```python
from build123d import *

# Parameters (mm, degrees)
F0_R      = 5.5120501068
F1_DEPTH  = 50
F3_DEPTH  = 13
F4_R      = 10
F5_DEPTH  = 7
F6_R      = 5
F7_DEPTH  = 6
F8_R      = 5.5120501068
F9_DEPTH  = 9
F11_DEPTH = 381
F13_DEPTH = 381
F14_W     = 50
F14_H     = 12
F15_DEPTH = 15
F16_R     = 5
F17_DEPTH = 381


with BuildPart() as f1:
    # F0 (on Front) → F1 (new body)
    with BuildSketch(Plane.XZ):
        with BuildLine():
            Line((60, -15), (60, 0))
            Line((60, 0), (0, 0))
            Line((0, 0), (0, -63))
            Line((0, -63), (45, -63))
            Line((45, -63), (72.4561188247, -53.0067899993))
            ThreePointArc((72.4561188247, -53.0067899993), (74.5109412295, -53.1845320084), (76.2667195414, -54.2667195414))
            Line((76.2667195414, -54.2667195414), (85, -63))
            Line((85, -63), (100, -63))
            Line((100, -63), (100, -15))
            Line((100, -15), (60, -15))
        make_face()
        with Locations((90, -28)):
            Circle(F0_R, mode=Mode.SUBTRACT)
    extrude(amount=F1_DEPTH)

    # F2 (on face) → F3 (cut)
    with BuildSketch(Plane.XZ.offset(50)):
        with BuildLine():
            Line((30, 0), (0, 0))
            Line((0, 0), (0, -50.6242252886))
            ThreePointArc((0, -50.6242252886), (11.1042474662, -53.9150696691), (22.5, -51.8484800354))
            ThreePointArc((22.5, -51.8484800354), (54.7104431454, -31.7939424821), (30, -3))
            Line((30, -3), (30, 0))
        make_face()
    extrude(amount=-F3_DEPTH, mode=Mode.SUBTRACT)

    # F4 (on face) → F5 (join)
    with BuildSketch(Plane.XZ.offset(37)):
        with Locations((30, -28)):
            Circle(F4_R)
    extrude(amount=F5_DEPTH)

    # F6 (on face) → F7 (join)
    with BuildSketch(Plane.XZ.offset(44)):
        with Locations((30, -28)):
            Circle(F6_R)
    extrude(amount=F7_DEPTH)

    # F8 (on face) → F9 (cut)
    with BuildSketch(Plane.XZ.offset(50)):
        with BuildLine():
            Line((100, -15), (80, -15))
            Line((80, -15), (80, -28))
            ThreePointArc((80, -28), (85.8578643763, -42.1421356237), (100, -48))
            Line((100, -48), (100, -15))
        make_face()
        with Locations((90, -28)):
            Circle(F8_R, mode=Mode.SUBTRACT)
    extrude(amount=-F9_DEPTH, mode=Mode.SUBTRACT)

    # F10 (on face) → F11 (cut)
    with BuildSketch(Plane.XZ.offset(50)):
        with BuildLine():
            Line((30, 0), (0, 0))
            Line((0, 0), (0, -56.8121126443))
            ThreePointArc((0, -56.8121126443), (21.1383307761, -48.7974627961), (30, -28))
            Line((30, -28), (30, 0))
        make_face()
    extrude(amount=-F11_DEPTH, mode=Mode.SUBTRACT)

    # F12 (on face) → F13 (cut)
    with BuildSketch(Plane(origin=(30, 0, 0), x_dir=(0, -1, 0), z_dir=(-1, 0, 0))):
        Polygon((6.5514642168, 0), (0, 0), (0, -18), align=None)
    extrude(amount=-F13_DEPTH, mode=Mode.SUBTRACT)

    # F14 (on Top) → F15 (cut)
    with BuildSketch(Plane.XY):
        with Locations((75.5128398538, -6)):
            Rectangle(F14_W, F14_H)
    extrude(amount=-F15_DEPTH, mode=Mode.SUBTRACT)

    # F16 (on face) → F17 (cut)
    with BuildSketch(Plane.XY):
        with Locations((39, -20)):
            Circle(F16_R)
    extrude(amount=-F17_DEPTH, mode=Mode.SUBTRACT)


solid = f1.part
```
Geometry check sheet. Reference: the model listing, model coordinates, mm. A direction names the side the tool comes from. Round coordinates to 2 decimals unless told otherwise and drop trailing zeros. Order: outer loops, then holes, each group sorted by start corner. A loop starts at its lowest first (then second) coordinate and runs counter-clockwise, first axis right, second up. Notation, with made-up numbers: (14.25, -22.5) - (55.25, -22.5) arc R32 cw to (55.25, 14.5) - close; hole circle Ø10 at (-29, -40). An arc over 180 degrees is marked (long way). Use a Markdown table: item, result. Add a question column.
1) Mould release check, pull along Y, two halves, no side actions. Record for faces 1 (the flat face through (35.4, -44, -27.9)), 2 (the cylindrical face through (35, -23, -31)), 3 (the flat face through (45, -28, 0)): released by +Y, released by -Y, zero draft, split by the parting line, or undercut.
2) Section check C-C (z = -42.5). Record the cut outline in (x, y), then the cut area to 3 significant figures.
3) Thickness scan on line 1 along Z through (x, y) = (90, -13); line 2 along Y through (x, z) = (39, -37.5); line 3 along X through (y, z) = (-19, -31). Record the ranges inside material, lowest first.
4) Section check D-D (x = 52). Record the cut outline in (y, z), then the cut area to 3 significant figures.
5) Section check B-B (x = 90). Record the cut outline in (y, z).
6) Gauge pin test, flat ends, axial feed: P1, Ø5.5, axis at y = -8.5, z = -8.5, coming from the +X side; P2, Ø3, axis at x = 55, z = -9.5, coming from the +Y side; P3, Ø7.5, axis at y = -32.5, z = -9, coming from the +X side. Record the tip position at first contact, or that the pin passes through.
7) Set-up check for faces 4 (the flat face through (39, -37, -34)), 5 (the flat face through (55, -12, -7)), 6 (the flat face through (81, -25, -59)), 7 (the cylindrical face through (18.186, -43.591, -53.288)): record each of +Z, -Z, +X, -X, +Y, -Y from which the full face is reachable in a straight line by a thin tool's end or side.
8) Section check A-A (y = -20). Record the cut outline in (x, z).
Established:
| question | item | result |
|---|---|---|
| 1 | face 1 | released by -Y |
| 1 | face 2 | undercut |
| 1 | face 3 | zero draft |
| 2 | outline | (26.09, -37) - (50.37, -37) - (50.37, -50) - (86.23, -50) - (86.23, -41) - (100, -41) - (100, 0) - (26.09, 0) - close; hole circle Ø10 at (39, -20) |
| 2 | area | 3,180 mm2 |
| 3 | line 1 | -63 to -33.51, -22.49 to -15 |
| 3 | line 2 | -37 to -25, -15 to 0 |
| 3 | line 3 | 29.84 to 34.1, 43.9 to 85.38, 94.62 to 100 |
| 4 | outline | (-50, -60.45) - (0, -60.45) - (0, -18) - (-1.09, -15) - (-12, -15) - (-12, 0) - (-50, 0) - (-50, -16.13) - (-37, -16.13) - (-37, -39.87) - (-50, -39.87) - close |
| 4 | area | 2,530 mm2 |
| 5 | outline | (-50, -63) - (0, -63) - (0, -33.51) - (-41, -33.51) - (-41, -45.32) - (-50, -45.32) - close; (-41, -22.49) - (0, -22.49) - (0, -18) - (-1.09, -15) - (-41, -15) - close |
| 6 | P1 | x = 50.51 |
| 6 | P2 | y = -12 |
| 6 | P3 | x = 60 |
| 7 | face 4 | -Y |
| 7 | face 5 | +Z, +X, +Y |
| 7 | face 6 | -Z, +Y, -Y |
| 7 | face 7 | +Z, -X, -Y |
| 8 | outline | (0, -63) - (34, -63) - (34, 0) - (30, 0) - (30, -28) arc R28.84 cw to (0, -56.81) - close; (44, -63) - (45, -63) - (72.46, -53.01) arc R4.47 cw to (76.27, -54.27) - (85, -63) - (100, -63) - (100, -15) - (60, -15) - (60, 0) - (44, 0) - close; hole circle Ø11.02 at (90, -28) |
